from build123d import *

# Parameters (mm, degrees)
SKETCH_1_R      = 1.7
EXTRUDE_1_DEPTH = 5


with BuildPart() as part:
    # 草图1 → 凸台-拉伸1 (new body)
    with BuildSketch(Plane(origin=(0, 0, 0), x_dir=(1, 0, 0), z_dir=(0, 1, 0))):
        Polygon((1439.011595349, 1417.863209963), (1439.011595349, 1369.863209963), (1433.011595349, 1363.863209963), (1415.011595349, 1363.863209963), (1409.011595349, 1369.863209963), (1409.011595349, 1417.863209963), (1416.08266316, 1424.934277775), (1431.940527537, 1424.934277775), align=None)
        with Locations(Location((1429.211595349, 1369.163209963, 0), (0, 0, 270))):
            Circle(SKETCH_1_R, mode=Mode.SUBTRACT)
        with Locations(Location((1419.211595349, 1369.163209963, 0), (0, 0, 270))):
            Circle(SKETCH_1_R, mode=Mode.SUBTRACT)
        with BuildLine():
            Line((1434.411595349, 1413.863209963), (1434.411595349, 1373.463209963))
            Line((1434.411595349, 1373.463209963), (1414.011595349, 1373.463209963))
            Line((1414.011595349, 1373.463209963), (1414.011595349, 1413.863209963))
            Line((1414.011595349, 1413.863209963), (1418.011595349, 1413.863209963))
            Line((1418.011595349, 1413.863209963), (1419.530084528, 1416.493310372))
            ThreePointArc((1419.530084528, 1416.493310372), (1417.739352162, 1419.013209963), (1420.817015405, 1418.722340038))
            Line((1420.817015405, 1418.722340038), (1422.011595349, 1420.791413193))
            Line((1422.011595349, 1420.791413193), (1426.411595349, 1420.791413193))
            Line((1426.411595349, 1420.791413193), (1427.606175292, 1418.722340038))
            ThreePointArc((1427.606175292, 1418.722340038), (1430.683838535, 1419.013209963), (1428.893106169, 1416.493310372))
            Line((1428.893106169, 1416.493310372), (1430.411595349, 1413.863209963))
            Line((1430.411595349, 1413.863209963), (1434.411595349, 1413.863209963))
        make_face(mode=Mode.SUBTRACT)
    extrude(amount=EXTRUDE_1_DEPTH)


solid = part.part
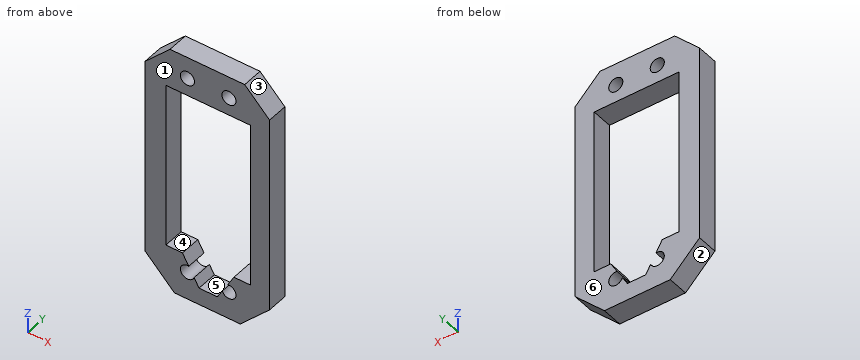
Source: CAD feature listing. Evaluate the final solid. Frame: model axes, mm. Face numbers are marked on the shaded views. A direction names the side the tool comes from. Round coordinates to 2 decimals unless told otherwise and drop trailing zeros. Loops run counter-clockwise (first coordinate to the right, second up) from the corner with the lowest first, then second, coordinate; pieces in that order, holes last. Notation, with made-up numbers: (-40, 75.5) - (-1, 75.5) arc R32 ccw to (-1, 112.5) - close; hole circle Ø2 at (57.5, -10). An arc over 180 degrees is marked (long way). Write item = value, one per line. Start each with the question number.
(1) Pull-direction query (X, two-part tool) for the marked faces 1, 2, 3 and 4; classes: +X half, -X half, draft (parallel to the pull), parting line (faces both ways), or undercut.
(2) Set-up query: the marked faces 5 and 6. Return all of +Z, -Z, +X, -X, +Y, -Y with unobstructed straight access to the full face (end or side cutting, diameter ignored); none if empty.
(3) Section query A-A, the plane z = -1398. Output: boundary loops of the cut face in (x, y), plus the area to 3 significant figures.
(4) Section query C-C, the plane x = 1420.25. Output: boundary loops of the cut face in (y, z).
(5) Section query D-D, the plane z = -1415. Output: boundary loops of the cut face in (x, y), plus the area to 3 significant figures.
(6) Section query B-B, the plane y = 1.65. Output: boundary loops of the cut face in (x, z), plus the area to 3 significant figures.
(7) Ray query, line 1 along X through (y, z) = (1, -1384); line 2 along Z through (x, y) = (1424.25, 1.65); line 3 along Z through (x, y) = (1428, 0.4). Return the intervals inside material, ascending. Write a range as from..to.
Conclusion:
q1.face_1 = draft
q1.face_2 = -X half
q1.face_3 = +X half
q1.face_4 = undercut
q2.face_5 = +Y, -Y
q2.face_6 = +Z, -Z, +X, -X, +Y
q3.outline = (1409.01, 0) - (1414.01, 0) - (1414.01, 5) - (1409.01, 5) - close; (1434.41, 0) - (1439.01, 0) - (1439.01, 5) - (1434.41, 5) - close
q3.area = 48.0 mm2
q4.outline = (0, -1424.93) - (5, -1424.93) - (5, -1419.51) - (0, -1419.51) - close; (0, -1373.46) - (5, -1373.46) - (5, -1370.51) - (0, -1370.51) - close; (0, -1367.82) - (5, -1367.82) - (5, -1363.86) - (0, -1363.86) - close
q5.outline = (1409.01, 0) - (1418.67, 0) - (1418.67, 5) - (1409.01, 5) - close; (1429.76, 0) - (1439.01, 0) - (1439.01, 5) - (1429.76, 5) - close
q5.area = 94.6 mm2
q6.outline = (1409.01, -1417.86) - (1416.08, -1424.93) - (1431.94, -1424.93) - (1439.01, -1417.86) - (1439.01, -1369.86) - (1433.01, -1363.86) - (1415.01, -1363.86) - (1409.01, -1369.86) - close; hole (1414.01, -1413.86) - (1418.01, -1413.86) - (1419.53, -1416.49) arc R1.7 ccw (long way) to (1420.82, -1418.72) - (1422.01, -1420.79) - (1426.41, -1420.79) - (1427.61, -1418.72) arc R1.7 ccw (long way) to (1428.89, -1416.49) - (1430.41, -1413.86) - (1434.41, -1413.86) - (1434.41, -1373.46) - (1414.01, -1373.46) - close; hole circle Ø3.4 at (1419.21, -1369.16); hole circle Ø3.4 at (1429.21, -1369.16)
q6.area = 830 mm2
q7.line_1 = 1409.01..1414.01, 1434.41..1439.01
q7.line_2 = -1424.93..-1420.79, -1373.46..-1363.86
q7.line_3 = -1424.93..-1419.36, -1373.46..-1370.36, -1367.97..-1363.86
